from build123d import *

# Parameters (mm, degrees)
F0_W     = 1070
F0_H     = 100
F1_DEPTH = 50
F2_T     = -4
F3_R     = 5
F5_D     = 22
F5_DEPTH = 4
F5_TIP   = 6.6094668093
F7_D     = 10
F7_DEPTH = 5
F7_TIP   = 3.0043030951


with BuildPart() as f1:
    # F0 (on Front) → F1 (new body)
    with BuildSketch(Plane.XZ):
        Rectangle(F0_W, F0_H)
    extrude(amount=F1_DEPTH)

    # F2
    f2_openings = [f1.faces().sort_by_distance(p)[0] for p in [
        (-535, -25, 0),
        (535, -25, 0),
    ]]
    offset(amount=F2_T, openings=f2_openings)

    # F3
    f3_edges = [f1.edges().sort_by_distance(p)[0] for p in [
        (0, -46, 46),
        (0, -4, 46),
        (0, -46, -46),
        (0, -4, -46),
        (0, -50, -50),
        (0, -50, 50),
        (0, 0, 50),
        (0, 0, -50),
    ]]
    fillet(f3_edges, radius=F3_R)

    # F5
    with Locations(Plane.XZ.offset(50)):
        with Locations((0, 0)):
            Hole(F5_D / 2, depth=F5_DEPTH)
            with Locations((0, 0, -(F5_DEPTH + F5_TIP / 2))):  # 118° drill point
                Cone(0, F5_D / 2, F5_TIP, mode=Mode.SUBTRACT)

    # F7
    with Locations(Plane(origin=(0, 0, 0), x_dir=(-1, 0, 0), z_dir=(0, 1, 0))):
        with Locations((238.0880117416, 0), (-238.088, 0)):
            Hole(F7_D / 2, depth=F7_DEPTH)
            with Locations((0, 0, -(F7_DEPTH + F7_TIP / 2))):  # 118° drill point
                Cone(0, F7_D / 2, F7_TIP, mode=Mode.SUBTRACT)


solid = f1.part
Verification items for the finished model (mm, model axes). A direction names the side the tool comes from. Give positions to 0.01 mm unless a question says otherwise; leave off trailing zeros. Write each loop counter-clockwise with the first axis right and the second up, starting at its lowest first coordinate (ties: lowest second). Pieces come first, ordered by that corner, then holes. Notation, with made-up numbers: M -13,31.5 L 42,31.5 A30 cw 42,60.5 Z; hole C 29.25,78 d3. An arc over 180 degrees is marked long. Use CSV: the item, a comma, the result in double quotes.
1) Access from +Z, -Z, +X, -X, +Y, -Y to the whole of each face (thin tool, end or side, straight path). Record for faces 1 (the face through (535, -47, 0)), 2 (the face through (-7, -46, 10)).
Final values:
face 1,"+Z, -Z, +X, +Y, -Y"
face 2,"+X, -X"
2) Cross-section at B-B (z = -22). Enter the section's corners in (x, y).
Final values:
outline,"M -535,-50 L 535,-50 L 535,-46 L -535,-46 Z; M -535,-4 L 535,-4 L 535,0 L -535,0 Z"
3) Release check for a two-part mould opening along X. For faces 3 (the face through (-535, -47, 0)), 4 (the face through (-7, 0, 1)), 5 (the face through (2.38, -47.97, -10.74)) record: released by +X, released by -X, zero draft, split by the parting line, or undercut.
Final values:
face 3,"released by -X"
face 4,"zero draft"
face 5,"undercut"
4) Cross-section at C-C (x = 163). Enter the section's corners in (y, z), plus the area to 3 significant figures.
Final values:
outline,"M -50,-45 A5 ccw -45,-50 L -5,-50 A5 ccw 0,-45 L 0,45 A5 ccw -5,50 L -45,50 A5 ccw -50,45 Z; hole M -46,-41 A5 ccw -41,-46 L -9,-46 A5 ccw -4,-41 L -4,41 A5 ccw -9,46 L -41,46 A5 ccw -46,41 Z"
area,"1,140 mm²"
5) Cross-section at A-A (y = -30). Enter the section's corners in (x, z).
Final values:
outline,"M -535,-50 L 535,-50 L 535,-46 L -535,-46 Z; M -535,46 L 535,46 L 535,50 L -535,50 Z"
6) Material ranges on line 1 along Z through (x, y) = (-117, -25); line 2 along Y through (x, z) = (-192, 22.5); line 3 along Z through (x, y) = (-308, -42.5), recorded low to high.
Final values:
line 1,"-50 to -46, 46 to 50"
line 2,"-50 to -46, -4 to 0"
line 3,"-50 to -45.77, 45.77 to 50"
7) Cross-section at D-D (x = 0). Enter the section's corners in (y, z), plus the area to 3 significant figures.
Final values:
outline,"M -50,-45 A5 ccw -45,-50 L -5,-50 A5 ccw 0,-45 L 0,45 A5 ccw -5,50 L -45,50 A5 ccw -50,45 L -50,11 L -46,11 L -46,41 A5 cw -41,46 L -9,46 A5 cw -4,41 L -4,-41 A5 cw -9,-46 L -41,-46 A5 cw -46,-41 L -46,-11 L -50,-11 Z"
area,"1,050 mm²"
8) Go/stop test with a flat-tipped pin: pin 1 Ø16 at (x, z) = (-238.09, 0) entering from +Y. Record where the tip stops, or that it passes through.
Final values:
pin 1,"y = 0"
